Geometry: final body of the model. Coordinates: model frame, mm. Face numbers are marked on the shaded views. A direction names the side the tool comes from. Round coordinates to 2 decimals unless told otherwise and drop trailing zeros. Order: outer loops, then holes, each group sorted by start corner. A loop starts at its lowest first (then second) coordinate and runs counter-clockwise, first axis right, second up. Notation, with made-up numbers: M -38,-0.75 L -4,-0.75 A19 cw -4,13.25 Z; hole C 47.25,48.25 d11. An arc over 180 degrees is marked long. Put each result on its own line as item: value. Start each with the question number.
1) Access query for the marked faces 4 and 5. Directions: +Z, -Z, +X, -X, +Y, -Y. A direction counts if a zero-diameter tool reaches every point of the face in a straight line with its end or side. Return the directions, or none.
2) Material intervals for probe 1 along Y at (x, z) = (-3, 0); probe 2 along X at (y, z) = (13, -9.5) (3 decimals); probe 3 along Y at (x, z) = (8, -4), sorted ascending. Write a range as [from, to].
3) Draft query along X for the marked faces 1, 2 and 3. Return one class per face: pulls with the +X half, pulls with the -X half, needs draft (parallel to the pull), parting line crosses it, or undercut.
4) First-contact query: P1, Ø10, axis at y = 0, z = 0, coming from the -X side; P2, Ø2, axis at x = 1.5, y = -4, coming from the -Z side; P3, Ø3, axis at x = -2, y = 2.5, coming from the -Z side; P4, Ø4, axis at x = 5, y = -2, coming from the +Z side. Flat tips, straight axial feed; report the tip coordinate or a pass-through.
5) Section A-A, the plane z = 0. Return loops of the section in (x, y) (3 decimals).
6) Section C-C, the plane x = 2.5. Return loops of the section in (y, z), then the cut area to 3 significant figures.
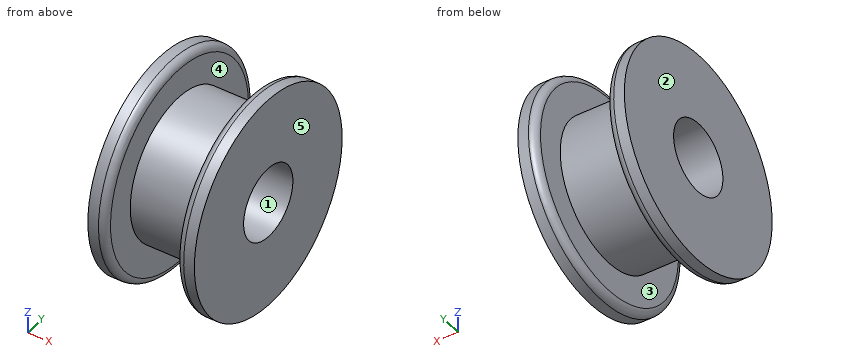
from build123d import *

# Parameters (mm, degrees)
SKETCH1_R            = 12.7
BOSS_EXTRUDE1_DEPTH  = 6.35
SKETCH2_R            = 19.05
BOSS_EXTRUDE2_DEPTH  = 3.175
FILLET1_R            = 1.27
FILLET1_OF_MIRROR1_R = 1.27
CUT_EXTRUDE1_REACH   = 21.05
SKETCH3_R            = 6.35


with BuildPart() as part:
    # Sketch1 → Boss-Extrude1 (new body)
    with BuildSketch(Plane(origin=(0, 0, 0), x_dir=(0, 0, -1), z_dir=(1, 0, 0))):
        Circle(SKETCH1_R)
    boss_extrude1 = extrude(amount=BOSS_EXTRUDE1_DEPTH)

    # Sketch2 → Boss-Extrude2 (add)
    with BuildSketch(Plane(origin=(6.35, 0, 0), x_dir=(0, 0, -1), z_dir=(1, 0, 0))):
        Circle(SKETCH2_R)
    boss_extrude2 = extrude(amount=BOSS_EXTRUDE2_DEPTH)

    # Fillet1
    fillet1_edges = [part.edges().sort_by_distance(p)[0] for p in [
        (6.35, 0, 19.05),
    ]]
    fillet(fillet1_edges, radius=FILLET1_R)

    # Mirror1: Boss-Extrude1, Boss-Extrude2 across plane
    add(boss_extrude1.mirror(Plane(origin=(0, 0, 0), x_dir=(0, 0, 1), z_dir=(1, 0, 0))))
    add(boss_extrude2.mirror(Plane(origin=(0, 0, 0), x_dir=(0, 0, 1), z_dir=(1, 0, 0))))

    # Fillet1 of Mirror1
    fillet1_of_mirror1_edges = [part.edges().sort_by_distance(p)[0] for p in [
        (-6.35, 0, 19.05),
    ]]
    fillet(fillet1_of_mirror1_edges, radius=FILLET1_OF_MIRROR1_R)

    # Sketch3 → Cut-Extrude1 (cut, up to next)
    with BuildSketch(Plane(origin=(9.525, 0, 0), x_dir=(0, 0, -1), z_dir=(1, 0, 0)), mode=Mode.PRIVATE) as cut_extrude1_sk1:
        Circle(SKETCH3_R)
    cut_extrude1_tool1 = extrude(cut_extrude1_sk1.sketch, amount=-CUT_EXTRUDE1_REACH, mode=Mode.PRIVATE) & part.part
    add(cut_extrude1_tool1.solids().sort_by_distance((9.525, 0, 0))[0], mode=Mode.SUBTRACT)


solid = part.part
Result sheet:
1. face 4: none
1. face 5: +Z, -Z, +X, +Y, -Y
2. probe 1: y = [-12.7, -6.35], [6.35, 12.7]
2. probe 2: x = [-9.525, -6.35], [6.35, 9.525]
2. probe 3: y = [-18.63, -4.93], [4.93, 18.63]
3. face 1: needs draft
3. face 2: pulls with the -X half
3. face 3: undercut
4. P1: passes through
4. P2: stops at z = -12.34
4. P3: stops at z = -12.66
4. P4: stops at z = 18.8
5. outline: M -9.525,-19.05 L -7.62,-19.05 A1.27 ccw -6.35,-17.78 L -6.35,-12.7 L 6.35,-12.7 L 6.35,-17.78 A1.27 ccw 7.62,-19.05 L 9.525,-19.05 L 9.525,-6.35 L -9.525,-6.35 Z; M -9.525,6.35 L 9.525,6.35 L 9.525,19.05 L 7.62,19.05 A1.27 ccw 6.35,17.78 L 6.35,12.7 L -6.35,12.7 L -6.35,17.78 A1.27 ccw -7.62,19.05 L -9.525,19.05 Z
6. outline: C 0,0 d25.4; hole C 0,0 d12.7
6. area: 380 mm2
